Autodesk Inventor part; units mm, degrees
ref_plane "YZ Plane" through (0, 0, 0) normal (1, 0, 0) x (0, 1, 0)
ref_plane "XZ Plane" through (0, 0, 0) normal (0, 1, 0) x (-1, 0, 0)
ref_plane "XY Plane" through (0, 0, 0) normal (0, 0, 1) x (1, 0, 0)
sketch "Sketch1" plane through (0, 0, 0) normal (0, 0, 1) x (1, 0, 0)
  line L0 (0, 0) -> (152.4, 0)
  line L1 (152.4, 0) -> (152.4, 120.65)
  line L2 (152.4, 120.65) -> (0, 120.65)
  line L3 (0, 120.65) -> (0, 0)
  dimension "d0" = 152.4
  dimension "d1" = 120.65
extrude "Extrusion1" add sketch "Sketch1" along normal blind 6.35
sketch "Sketch2" plane through (0, 0, 6.35) normal (0, 0, 1) x (1, 0, 0)
  line L0 (0, 0) -> (152.4, 0)
  line L1 (152.4, 120.65) -> (0, 120.65)
  line L2 (114.2866, 59.261) -> (0, 60.6355)
  line L3 (0, 120.65) -> (0, 0)
  line L4 (76.2, 0) -> (76.2, 120.65)
  circle A0 centre (25.4, 25.4) radius 3.175
  circle A1 centre (26.2401, 95.25) radius 3.175
  point P0 (114.7072, 94.0562)
  dimension "d18" = 25.4
  dimension "d20" = 25.4
  dimension "d23" = 25.4
  dimension "d24" = 26.2401
  dimension "d31" = 69.85
  dimension "d32" = 6.35
sketch "Sketch3" plane through (0, 0, 6.35) normal (0, 0, 1) x (1, 0, 0)
  point P0 (0, 0)
extrude "Extrusion4" add sketch "Sketch2" along normal blind 19.05 contours A0 | A1
thread "Thread5"
thread "Thread6"
sketch "Sketch7" plane through (0, 0, 0) normal (0, 0, -1) x (-1, 0, 0)
  line L0 (-152.4, 0) -> (-152.4, 120.65)
  line L1 (0, 0) -> (-152.4, 0)
  line L2 (-152.4, 120.65) -> (-142.875, 120.65)
  line L3 (-142.875, 120.65) -> (-142.875, 0)
  line L4 (-142.875, 0) -> (-152.4, 0)
  line L5 (-152.4, 0) -> (-152.4, 120.65)
  dimension "d36" = 9.525
extrude "Extrusion6" add sketch "Sketch7" along normal blind 63.5
sketch "Sketch8" plane through (152.4, 0, 6.35) normal (1, 0, 0) x (0, 0, -1)
  line L0 (69.85, 0) -> (69.85, 120.65)
  line L1 (0, 0) -> (0, 120.65)
  line L2 (69.85, 107.95) -> (34.29, 95.5609)
  line L3 (34.29, 95.5609) -> (34.29, 19.05)
  line L4 (34.29, 19.05) -> (69.85, 6.35)
  point P0 (6.35, 0)
  point P1 (34.29, 108.2609)
  point P2 (34.29, 6.35)
  dimension "d39" = 12.7
  dimension "d40" = 12.7
  dimension "d41" = 34.29
  dimension "d42" = 34.29
  dimension "d43" = 34.29
  dimension "d44" = 34.29
extrude "Extrusion7" cut sketch "Sketch8" against normal blind 63.5
fillet "Fillet1" radius 3.175 5 edges at (147.6375, 120.65, -63.5) (147.6375, 107.95, -63.5) (147.6375, 95.5609, -27.94) (147.6375, 19.05, -27.94) (147.6375, 6.35, -63.5)
properties part number "LucasCharles Part 10 final" material "Stainless Steel, Austenitic"
Geometry check sheet. Reference: the model listing, model coordinates, mm. A direction names the side the tool comes from. Give positions to 0.01 mm unless a question says otherwise; leave off trailing zeros. Write each loop counter-clockwise with the first axis right and the second up, starting at its lowest first coordinate (ties: lowest second). Pieces come first, ordered by that corner, then holes.
1) Section check C-C, the plane z = -18. Record the boundary of the cut face in (x, y) (3 decimals), and give its area (3 significant figures).
2) Gauge pin test, flat ends, axial feed: pin 1 (19 mm diameter, centred on y = 77, z = -27, fed in from -X) (3 decimals); pin 2 (10 mm diameter, centred on y = 32.5, z = 1.5, fed in from -X); pin 3 (3 mm diameter, centred on x = 149.5, y = 61.5, fed in from -Z); pin 4 (4 mm diameter, centred on x = 90, y = 39.5, fed in from -Z). Record the tip position at first contact, or that the pin passes through.
3) Material ranges on L1, parallel to X at y = 43, z = -7.5 (3 decimals); L2, parallel to Z at x = 29, y = 34; L3, parallel to Y at x = 145.5, z = -57, recorded low to high.
4) Section check D-D, the plane x = 25.4. Record the boundary of the cut face in (y, z) (3 decimals), and give its area (3 significant figures).
5) Section check B-B, the plane z = 20. Record the boundary of the cut face in (x, y) (3 decimals).
6) Section check A-A, the plane y = 52.5. Record the boundary of the cut face in (x, z) (3 decimals), and give its area (3 significant figures).
7) Access from +Z, -Z, +X, -X, +Y, -Y to the whole of each face (thin tool, end or side, straight path). Record for faces 1 (the flat face through (148, 114, -63.5)), 2 (the flat face through (110.4, 120.65, 0.3)), 3 (the cylindrical face through (28.43, 24.45, 15.74)), 4 (the flat face through (142.875, 61, -24)), 5 (the flat face through (147.7, 101.83, -45.94)).
8) Release check for a two-part mould opening along Y. For faces 6 (the flat face through (147.7, 12.78, -45.5)), 7 (the flat face through (110, 0, 3)), 8 (the flat face through (25, 25, 25.4)) record: pulls with the +Y half, pulls with the -Y half, needs draft (parallel to the pull), parting line crosses it, or undercut.
Computed:
1. outline: (142.875, 0) - (152.4, 0) - (152.4, 120.65) - (142.875, 120.65) - close
1. area: 1,150 mm2
2. pin 1: stops at x = 142.875
2. pin 2: stops at x = 0
2. pin 3: stops at z = -27.94
2. pin 4: stops at z = 0
3. L1: x = 142.875 to 152.4
3. L2: z = 0 to 6.35
3. L3: y = 0 to 8.67, 105.69 to 120.65
4. outline: (0, 0) - (120.65, 0) - (120.65, 6.35) - (98.312, 6.35) - (98.312, 25.4) - (92.188, 25.4) - (92.188, 6.35) - (28.575, 6.35) - (28.575, 25.4) - (22.225, 25.4) - (22.225, 6.35) - (0, 6.35) - close
4. area: 1,000 mm2
5. outline: circle Ø6.35 at (25.4, 25.4); circle Ø6.35 at (26.24, 95.25)
6. outline: (0, 0) - (142.875, 0) - (142.875, -27.94) - (152.4, -27.94) - (152.4, 6.35) - (0, 6.35) - close
6. area: 1,230 mm2
7. face 1: -Z, +X, -X, +Y, -Y
7. face 2: +Z, -Z, +X, -X, +Y
7. face 3: +Z
7. face 4: -Z, -X, +Y, -Y
7. face 5: -Z, +X, -X
8. face 6: undercut
8. face 7: pulls with the -Y half
8. face 8: needs draft
